Geometry check sheet. Reference: the model listing, model coordinates, mm. Face numbers are marked on the shaded views. Give positions to 0.01 mm unless a question says otherwise; leave off trailing zeros. Order: outer loops, then holes, each group sorted by start corner. A loop starts at its lowest first (then second) coordinate and runs counter-clockwise, first axis right, second up. Notation, with made-up numbers: M 18.25,1.25 L 56.25,1.25 A9 ccw 56.25,13.25 Z; hole C -34.75,65.5 d11. An arc over 180 degrees is marked long. Put each result on its own line as item: value. Start each with the question number.
Q1. Section check A-A on y = -10. Record the cut outline in (x, z), then the cut area to 3 significant figures.
Q2. Material ranges on L1, parallel to Y at x = 29.25, z = 15.25; L2, parallel to Z at x = 35.5, y = -10; L3, parallel to Y at x = 38.25, z = 16, recorded low to high.
Q3. Section check B-B on x = 30.75. Record the cut outline in (y, z), then the cut area to 3 significant figures.
Q4. Go/stop test with flat-tipped pins: pin 1 (3 mm diameter, centred on x = 38, z = 13.5, fed in from -Y); pin 2 (5 mm diameter, centred on x = 38.5, z = 11.5, fed in from -Y); pin 3 (5.5 mm diameter, centred on y = -10, z = 15.37, fed in from +X). Record where each tip stops, or that it passes through.
Q5. Mould release check, pull along Z, two halves, no side actions. Record for the marked faces 1, 2 and 3: +Z half, -Z half, draft (parallel to the pull), parting line (faces both ways), or undercut.
Q6. Section check C-C on z = 13.5. State how many separate pieces and enclosed holes the cut face has, then the cut area to 3 significant figures.
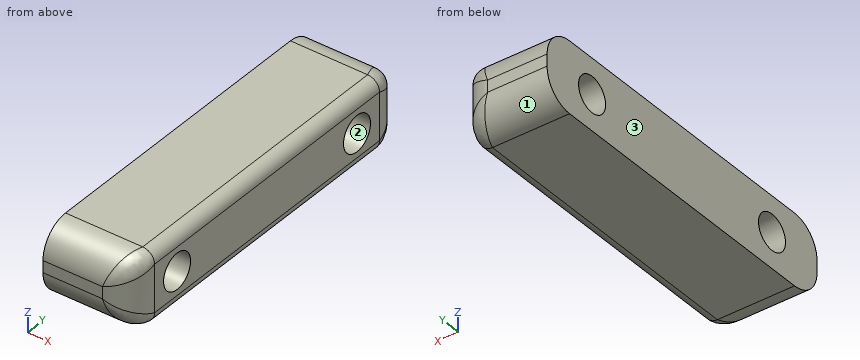
```python
from build123d import *

# Parameters (mm, degrees)
SKETCH001_W = 12
SKETCH001_H = 60
SKETCH001_R = 3
PAD_DEPTH   = 15
FILLET_R    = 2
FILLET001_R = 2
FILLET002_R = 5
FILLET003_R = 5


with BuildPart() as part:
    # Sketch001 → Pad (new body)
    with BuildSketch(Plane(origin=(26.164927, 0, 0), x_dir=(0, 0, 1), z_dir=(1, 0, 0))):
        with Locations((15.367814, 30)):
            Rectangle(SKETCH001_W, SKETCH001_H)
        with Locations((15.367814, 10)):
            Circle(SKETCH001_R, mode=Mode.SUBTRACT)
        with Locations((15.367814, 50)):
            Circle(SKETCH001_R, mode=Mode.SUBTRACT)
    extrude(amount=PAD_DEPTH)

    # Fillet
    fillet_edges = [part.edges().sort_by_distance(p)[0] for p in [
        (41.164927, -30, 9.367814),
    ]]
    fillet(fillet_edges, radius=FILLET_R)

    # Fillet001
    fillet001_edges = [part.edges().sort_by_distance(p)[0] for p in [
        (41.164927, -30, 21.367814),
    ]]
    fillet(fillet001_edges, radius=FILLET001_R)

    # Fillet002
    fillet002_edges = [part.edges().sort_by_distance(p)[0] for p in [
        (41.164927, -60, 15.367814),
    ]]
    fillet(fillet002_edges, radius=FILLET002_R)

    # Fillet003
    fillet003_edges = [part.edges().sort_by_distance(p)[0] for p in [
        (41.164927, 0, 15.367814),
    ]]
    fillet(fillet003_edges, radius=FILLET003_R)


solid = part.part
```
Results found:
1. outline: M 26.16,9.37 L 39.16,9.37 A2 ccw 41.16,11.37 L 41.16,12.37 L 26.16,12.37 Z; M 26.16,18.37 L 41.16,18.37 L 41.16,19.37 A2 ccw 39.16,21.37 L 26.16,21.37 Z
1. area: 88.3 mm^2
2. L1: y = -60 to -53, -47 to -13, -7 to 0
2. L2: z = 9.37 to 12.37, 18.37 to 21.37
2. L3: y = -59.54 to -52.93, -47.07 to -12.93, -7.07 to -0.46
3. outline: M -60,14.37 A5 ccw -55,9.37 L -5,9.37 A5 ccw 0,14.37 L 0,16.37 A5 ccw -5,21.37 L -55,21.37 A5 ccw -60,16.37 Z; hole C -50,15.37 d6; hole C -10,15.37 d6
3. area: 642 mm^2
4. pin 1: stops at y = -59.98
4. pin 2: stops at y = -59.9
4. pin 3: passes through
5. face 1: -Z half
5. face 2: undercut
5. face 3: draft
6. separate pieces: 3
6. enclosed holes: 0
6. area: 747 mm^2
